Work out the finished part from the listing and answer in its coordinate system (mm). Face numbers are marked on the shaded views. A direction names the side the tool comes from. Round coordinates to 2 decimals unless told otherwise and drop trailing zeros. Write each loop counter-clockwise with the first axis right and the second up, starting at its lowest first coordinate (ties: lowest second). Pieces come first, ordered by that corner, then holes.
Autodesk Fusion 360 part; units mm, degrees
sketch "Sketch1" plane through (0, 0, 0) normal (0, 1, 0) x (1, 0, 0)
  line L0 (10, 10) -> (-10, 10)
  line L1 (-10, 10) -> (-10, -10)
  line L2 (-10, -10) -> (10, -10)
  line L3 (10, -10) -> (10, 10)
  line L4 (10, 10) -> (-10, -10) construction
  line L5 (-10, 10) -> (10, -10) construction
  circle A0 centre (-5, 0) radius 1.8
  circle A1 centre (5, 0) radius 1.8
  line L6 (-10, -10) -> (10, -10)
  line L7 (10, -10) -> (10, -26)
  line L8 (10, -26) -> (-10, -26)
  line L9 (-10, -26) -> (-10, -10)
  line L10 (10, -10) -> (-10, -26) construction
  line L11 (-10, -10) -> (10, -26) construction
  circle A2 centre (0, -18) radius 4.05
  dimension "d52" = 20
  dimension "d53" = 20
  dimension "d55" = 10
  dimension "d56" = 3.6
  dimension "d57" = 3.6
  dimension "d58" = 20
  dimension "d59" = 16
  dimension "d60" = 8.1
extrude "Extrude1" add sketch "Sketch1" against normal blind 10
extrude "Extrude2" add sketch "Sketch1" along normal blind 20 contours L2 L6 L7 L8 L9 | A2
sketch "Sketch2" plane through (0, 0, 26) normal (0, 0, 1) x (-1, 0, 0)
  line L0 (10, -20) -> (-10, -20)
  line L1 (-10, -20) -> (-10, 0)
  line L2 (-10, 0) -> (10, 0)
  line L3 (10, 0) -> (10, -20)
  line L4 (-10, 0) -> (10, -20) construction
  line L5 (10, 0) -> (-10, -20) construction
  circle A0 centre (5, -10) radius 1.8
  circle A1 centre (-5, -10) radius 1.8
  line L6 (10, -20) -> (10, 10)
  line L7 (10, 10) -> (-10, 10)
  line L8 (-10, 10) -> (-10, -20)
  line L9 (-10, -20) -> (10, -20)
  line L10 (10, 0) -> (-10, 10) construction
  line L11 (-10, 0) -> (10, 10) construction
  circle A2 centre (0, 5) radius 1.55
  circle A3 centre (-5, -10) radius 3
  circle A4 centre (5, -10) radius 3
  dimension "d65" = 20
  dimension "d66" = 20
  dimension "d68" = 10
  dimension "d69" = 3.6
  dimension "d70" = 3.6
  dimension "d82" = 3.1
  dimension "d89" = 6
  dimension "d90" = 6
extrude "Extrude6" cut sketch "Sketch2" against normal blind 16 contours A0 | A1
extrude "Extrude7" cut sketch "Sketch2" against normal blind 4.5 contours A2
fillet "Fillet2" radius 1 1 edges at (0, 0, 10)
extrude "Extrude8" cut sketch "Sketch2" against normal blind 6 contours A3 | A4
chamfer "Chamfer4" distance 1 angle 45 19 edges at (10, 20, 18) (10, 10.5, 10) (10, 0, -0.5) (10, 0.2929, 9.7071) (10, 5, 26) (0, 20, 26) (-10, 5, 26) (0, -10, 26) (10, -10, 8) (-10, 0, -0.5) (-10, 0.2929, 9.7071) (-10, 10.5, 10) (-10, 20, 18) (0, 20, 10) (0, 0, -10) (10, -5, -10) (-10, -5, -10) (0, -10, -10) (-10, -10, 8)
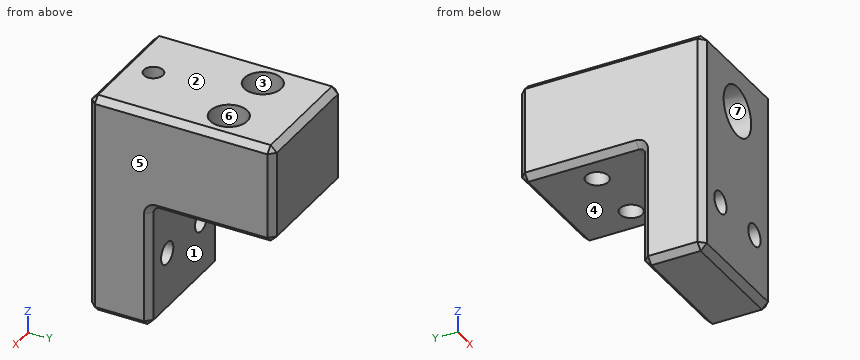
Q1. The mould has two halves that part along X. Classify the marked faces 4, 5, 6 and 7: +X half, -X half, draft (parallel to the pull), parting line (faces both ways), or undercut.
Q2. Find the intervals of material crossed by L1, parallel to X at y = 10, z = 22; L2, parallel to X at y = 10, z = 13.5; L3, parallel to Z at x = -5, y = -3, in increasing order.
Q3. Find section D-D (y = -5). Determine the outline of the cut face in (x, z), plus the area to 3 significant figures.
Q4. A tool of negligible diameter and unlimited length cuts with its end or side. For the marked faces 1, 2 and 3, from which of +Z, -Z, +X, -X, +Y, -Y can it reach the whole face along a straight path? Write none if from no direction.
Q5. Given pin 1 (4 mm diameter, centred on x = -5, z = 0, fed in from -Y); pin 2 (6.5 mm diameter, centred on x = 0, z = 18, fed in from -Y); pin 3 (2 mm diameter, centred on x = -4, y = 10.5, fed in from +Z); pin 4 (6 mm diameter, centred on x = 2, y = 16.5, fed in from -Z), each flat-ended and moving along its own axis, determine where each tip first touches the part or whether it passes through.
Q6. Find section A-A (z = 0). Determine the outline of the cut face in (x, y), plus the area to 3 significant figures.
Q7. Find section C-C (x = 0). Determine the outline of the cut face in (y, z).
Q8. Find section B-B (y = 10). Determine the outline of the cut face in (x, z).
Report:
1. face 4: draft
1. face 5: +X half
1. face 6: undercut
1. face 7: undercut
2. L1: x = -10 to -8, -2 to 2, 8 to 10
2. L2: x = -10 to -6.8, -3.2 to 3.2, 6.8 to 10
2. L3: z = -10 to -1.8, 1.8 to 26
3. outline: (-10, -9) - (-9, -10) - (9, -10) - (10, -9) - (10, 25) - (9, 26) - (1.55, 26) - (1.55, 21.74) arc R4.05 cw (long way) to (-1.55, 21.74) - (-1.55, 26) - (-9, 26) - (-10, 25) - close; hole circle Ø3.6 at (-5, 0); hole circle Ø3.6 at (5, 0)
3. area: 634 mm2
4. face 1: -Z, +X, -X, +Y
4. face 2: +Z, +X, -X, +Y, -Y
4. face 3: +Z
5. pin 1: stops at y = -10
5. pin 2: stops at y = 0
5. pin 3: stops at z = 20
5. pin 4: stops at z = 10
6. outline: (-10, -9) - (-9, -10) - (-6.8, -10) - (-6.8, 0) - (-9, 0) - (-10, -1) - close; (-3.2, -10) - (3.2, -10) - (3.2, 0) - (-3.2, 0) - close; (6.8, -10) - (9, -10) - (10, -9) - (10, -1) - (9, 0) - (6.8, 0) - close
6. area: 126 mm2
7. outline: (-10, -9) - (-9, -10) - (-1, -10) - (0, -9) - (0, 9) arc R1 cw to (1, 10) - (19, 10) - (20, 11) - (20, 25) - (19, 26) - (-3.45, 26) - (-3.45, 22.05) - (0, 22.05) - (0, 13.95) - (-10, 13.95) - close; (-10, 22.05) - (-6.55, 22.05) - (-6.55, 26) - (-9, 26) - (-10, 25) - close
8. outline: (-10, 11) - (-9, 10) - (-6.8, 10) - (-6.8, 20) - (-8, 20) - (-8, 26) - (-9, 26) - (-10, 25) - close; (-3.2, 10) - (3.2, 10) - (3.2, 20) - (2, 20) - (2, 26) - (-2, 26) - (-2, 20) - (-3.2, 20) - close; (6.8, 10) - (9, 10) - (10, 11) - (10, 25) - (9, 26) - (8, 26) - (8, 20) - (6.8, 20) - close
